Input: dimensioned drawing with shaded views. Units: mm. Origin: part minimum x, y, z. Round coordinates to 2 decimals unless told otherwise and drop trailing zeros. Loops run counter-clockwise (first coordinate to the right, second up) from the corner with the lowest first, then second, coordinate; pieces in that order, holes last. Notation, with made-up numbers: (62, 80.5) - (85, 80.5) arc R34 ccw to (85, 118.5) - close; hole circle Ø11 at (42.5, 37.5). An arc over 180 degrees is marked (long way). Answer as CSV lines item,"result".
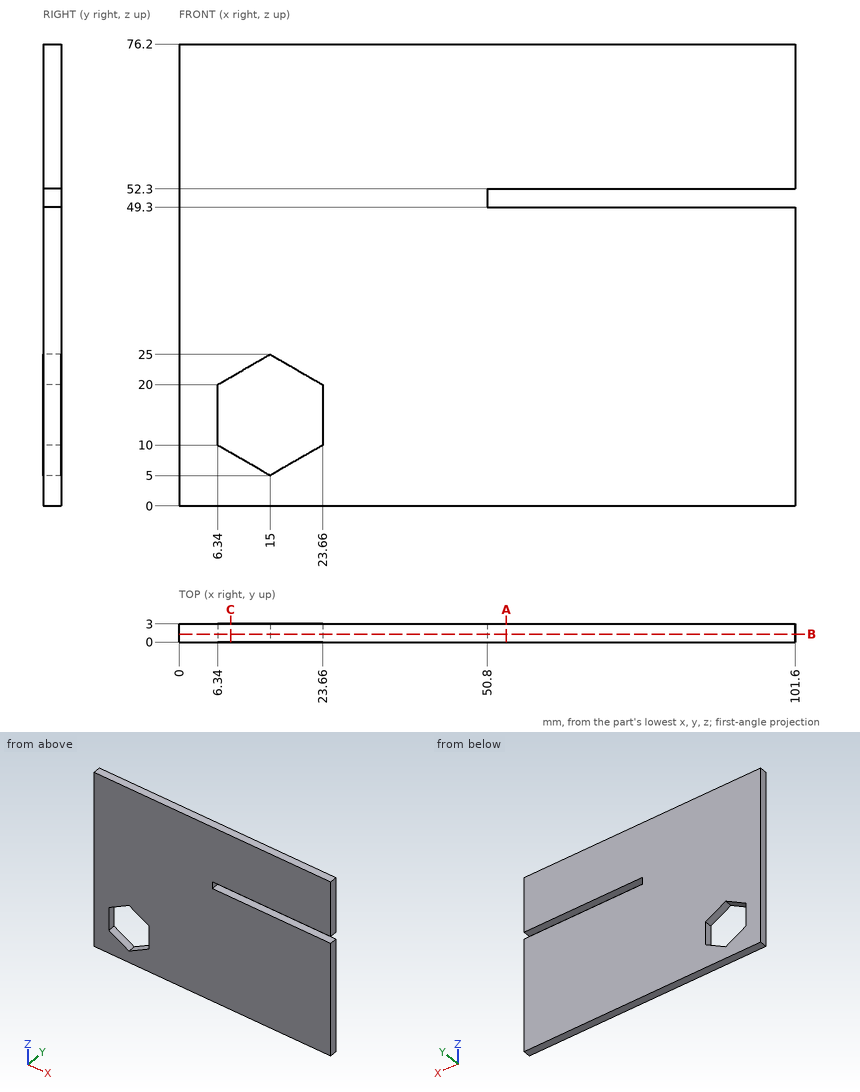
(1) Section A-A (x = 54). Output: boundary loops of the cut face in (y, z), and give its area (3 significant figures).
Findings below:
outline,"(0, 0) - (3, 0) - (3, 49.3) - (0, 49.3) - close; (0, 52.3) - (3, 52.3) - (3, 76.2) - (0, 76.2) - close"
area,"220 mm2"
(2) Section C-C (x = 8.5). Output: boundary loops of the cut face in (y, z).
Findings below:
outline,"(0, 0) - (3, 0) - (3, 8.75) - (0, 8.75) - close; (0, 21.25) - (3, 21.25) - (3, 76.2) - (0, 76.2) - close"
(3) Material intervals for line 1 along Z through (x, y) = (71.5, 1.05); line 2 along X through (y, z) = (2, 11); line 3 along X through (y, z) = (2.3, 8) (1 decimal), sorted ascending.
Findings below:
line 1,"0 to 49.3, 52.3 to 76.2"
line 2,"0 to 6.34, 23.66 to 101.6"
line 3,"0 to 9.8, 20.2 to 101.6"
(4) Pin query (flat end, axial travel): P1, Ø1.5, axis at y = 1.5, z = 51, coming from the +X side. Return the tip coordinate at first contact, or that it passes through.
Findings below:
P1,"x = 50.8"
(5) Section B-B (y = 1.3). Output: boundary loops of the cut face in (x, z), and give its area (3 significant figures).
Findings below:
outline,"(0, 0) - (101.6, 0) - (101.6, 49.3) - (50.8, 49.3) - (50.8, 52.3) - (101.6, 52.3) - (101.6, 76.2) - (0, 76.2) - close; hole (6.34, 10) - (15, 5) - (23.66, 10) - (23.66, 20) - (15, 25) - (6.34, 20) - close"
area,"7,330 mm2"
